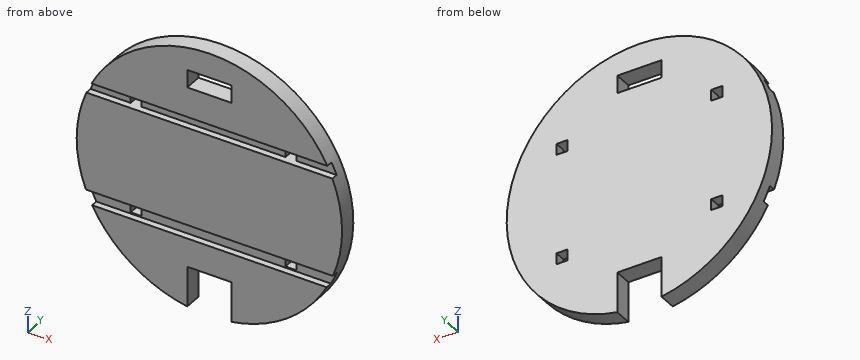
```python
from build123d import *

# Parameters (mm, degrees)
F0_R     = 60
F1_DEPTH = 8
F2_W     = 70
F2_H     = 2.5
F2_H_2   = 3.077762
F3_DEPTH = 3
F4_W     = 2.5
F4_H     = 2.5
F5_DEPTH = 8.001
F7_DEPTH = 8.001
F9_DEPTH = 8.001


with BuildPart() as f1:
    # F0 (on Front) → F1 (new body)
    with BuildSketch(Plane.XZ):
        Circle(F0_R)
    extrude(amount=F1_DEPTH)

    # F2 (on face) → F3 (cut)
    with BuildSketch(Plane.XZ.offset(8)):
        with BuildLine():
            Line((-35, 25), (35, 25))
            Line((35, 25), (35, 22.5))
            Line((35, 22.5), (55.621489, 22.5))
            ThreePointArc((55.621489, 22.5), (54.531492, 25.026314), (53.326823, 27.5))
            Line((53.326823, 27.5), (-53.326823, 27.5))
            ThreePointArc((-53.326823, 27.5), (-54.531492, 25.026314), (-55.621489, 22.5))
            Line((-55.621489, 22.5), (-35, 22.5))
            Line((-35, 22.5), (-35, 25))
        make_face()
        with Locations((0, 23.75)):
            Rectangle(F2_W, F2_H)
        with BuildLine():
            Line((55.851728, -21.922238), (35, -21.922238))
            Line((35, -21.922238), (35, -25))
            Line((35, -25), (-35, -25))
            Line((-35, -25), (-35, -21.922238))
            Line((-35, -21.922238), (-55.851728, -21.922238))
            ThreePointArc((-55.851728, -21.922238), (-54.525244, -25.039923), (-53.024893, -28.077762))
            Line((-53.024893, -28.077762), (53.024893, -28.077762))
            ThreePointArc((53.024893, -28.077762), (54.525244, -25.039923), (55.851728, -21.922238))
        make_face()
        with Locations((0, -23.461119)):
            Rectangle(F2_W, F2_H_2)
    extrude(amount=-F3_DEPTH, mode=Mode.SUBTRACT)

    # F4 (on face) → F5 (cut, through all)
    with BuildSketch(Plane.XZ.offset(8)):
        Polygon((-35, 25), (-32.5, 25), (-32.5, 27.5), (-37.5, 27.5), (-37.5, 22.5), (-35, 22.5), align=None)
        with Locations((-33.75, 23.75)):
            Rectangle(F4_W, F4_H)
        Polygon((32.5, 25), (35, 25), (35, 22.5), (37.5, 22.5), (37.5, 27.5), (32.5, 27.5), align=None)
        with Locations((33.75, 23.75)):
            Rectangle(F4_W, F4_H)
        Polygon((37.5, -22.5), (35, -22.5), (35, -25), (32.5, -25), (32.5, -27.5), (37.5, -27.5), align=None)
        with Locations((33.75, -23.75)):
            Rectangle(F4_W, F4_H)
        Polygon((-35, -25), (-35, -22.5), (-37.5, -22.5), (-37.5, -27.5), (-32.5, -27.5), (-32.5, -25), align=None)
        with Locations((-33.75, -23.75)):
            Rectangle(F4_W, F4_H)
    extrude(amount=-F5_DEPTH, mode=Mode.SUBTRACT)

    # F6 (on face) → F7 (cut, through all)
    with BuildSketch(Plane.XZ.offset(8)):
        Polygon((-10, 41), (0, 41), (10, 41), (10, 49), (-10, 49), align=None)
        Polygon((10, -41), (0, -41), (-10, -41), (-10, -49), (10, -49), align=None)
    extrude(amount=-F7_DEPTH, mode=Mode.SUBTRACT)

    # F8 (on face) → F9 (cut, through all)
    with BuildSketch(Plane(origin=(0, 0, 0), x_dir=(-1, 0, 0), z_dir=(0, 1, 0))):
        with BuildLine():
            Line((10, -49), (-10, -49))
            Line((-10, -49), (-10, -59.160798))
            ThreePointArc((-10, -59.160798), (0, -60), (10, -59.160798))
            Line((10, -59.160798), (10, -49))
        make_face()
    extrude(amount=-F9_DEPTH, mode=Mode.SUBTRACT)


solid = f1.part
```
Verification items for the finished model (mm, model axes). Coordinates: 2 decimals unless noted, no trailing zeros. Loops run counter-clockwise (first coordinate to the right, second up) from the corner with the lowest first, then second, coordinate; pieces in that order, holes last. Notation, with made-up numbers: (34, 74.25) -> (76, 74.25) arc R22 ccw to (76, 100.25) -> close; hole circle Ø10 at (-17.75, -15). An arc over 180 degrees is marked (long way). Put each result on its own line as item: value.
1. Gauge pin test, flat ends, axial feed: P1, Ø1.5, axis at y = -2.5, z = 25, coming from the -X side; P2, Ø4, axis at y = -2.5, z = -49.5, coming from the -X side; P3, Ø1.5, axis at y = -4, z = -43.5, coming from the -X side. Record the tip position at first contact, or that the pin passes through.
Result set:
P1: stops at x = -54.88
P2: stops at x = -36.66
P3: stops at x = -42.1
2. Section check D-D, the plane x = -29.5. Record the boundary of the cut face in (y, z).
Result set:
outline: (-8, -52.25) -> (0, -52.25) -> (0, 52.25) -> (-8, 52.25) -> (-8, 27.5) -> (-5, 27.5) -> (-5, 22.5) -> (-8, 22.5) -> (-8, -21.92) -> (-5, -21.92) -> (-5, -28.08) -> (-8, -28.08) -> close
3. Section check C-C, the plane z = 25. Record the boundary of the cut face in (x, y), then the cut area to 3 significant figures.
Result set:
outline: (-54.54, -5) -> (-37.5, -5) -> (-37.5, 0) -> (-54.54, 0) -> close; (-32.5, -5) -> (32.5, -5) -> (32.5, 0) -> (-32.5, 0) -> close; (37.5, -5) -> (54.54, -5) -> (54.54, 0) -> (37.5, 0) -> close
area: 495 mm^2
4. Thickness scan on line 1 (Z direction, x = -22.5, y = -5.75); line 2 (Z direction, x = 34, y = -3); line 3 (Z direction, x = -2, y = -0.75). Record the ranges inside material, lowest first.
Result set:
line 1: z = -55.62 to -28.08, -21.92 to 22.5, 27.5 to 55.62
line 2: z = -49.44 to -27.5, -22.5 to 22.5, 27.5 to 49.44
line 3: z = -41 to 41, 49 to 59.97
5. Section check A-A, the plane y = -6.5. Record the boundary of the cut face in (x, z).
Result set:
outline: (-55.85, -21.92) -> (55.85, -21.92) arc R60 ccw to (55.62, 22.5) -> (-55.62, 22.5) arc R60 ccw to start; (-53.33, 27.5) -> (53.33, 27.5) arc R60 ccw to start; (-53.02, -28.08) arc R60 ccw to (-10, -59.16) -> (-10, -41) -> (10, -41) -> (10, -59.16) arc R60 ccw to (53.02, -28.08) -> close; hole (-10, 41) -> (10, 41) -> (10, 49) -> (-10, 49) -> close
6. Section check B-B, the plane x = 0. Record the boundary of the cut face in (y, z).
Result set:
outline: (-8, -41) -> (0, -41) -> (0, 41) -> (-8, 41) -> (-8, 27.5) -> (-5, 27.5) -> (-5, 22.5) -> (-8, 22.5) -> (-8, -21.92) -> (-5, -21.92) -> (-5, -28.08) -> (-8, -28.08) -> close; (-8, 49) -> (0, 49) -> (0, 60) -> (-8, 60) -> close
